Input: part model. Units: mm. Frame: model coordinates. Give positions to 0.01 mm unless a question says otherwise; leave off trailing zeros. Loops run counter-clockwise (first coordinate to the right, second up) from the corner with the lowest first, then second, coordinate; pieces in that order, holes last. Notation, with made-up numbers: (67, -17) - (91, -17) arc R16 cw to (91, 11) - close; hole circle Ø2 at (16, 69.5). An arc over 180 degrees is marked (long way). One line per item, written item: value.
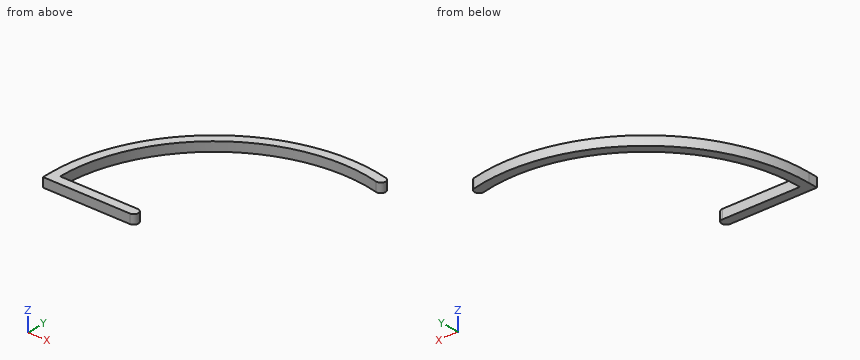
from build123d import *

# Parameters (mm, degrees)
BOSS_EXTRUDE1_DEPTH = 5


with BuildPart() as part:
    # Sketch1 → Boss-Extrude1 (new, symmetric)
    with BuildSketch(Plane.XY):
        with BuildLine():
            Line((552.821544179, 848.961112624), (459.088326812, 848.961112624))
            Line((459.088326812, 848.961112624), (459.088326812, 858.961112624))
            ThreePointArc((459.088326812, 858.961112624), (525.634918269, 996.884166681), (675.00895728, 1030.627523725))
            ThreePointArc((675.00895728, 1030.627523725), (678.753172827, 1024.629119776), (672.754768877, 1020.884904229))
            ThreePointArc((672.754768877, 1020.884904229), (531.858185738, 989.056590938), (469.088326812, 858.961112624))
            Line((469.088326812, 858.961112624), (552.821544179, 858.961112624))
            ThreePointArc((552.821544179, 858.961112624), (557.821544179, 853.961112624), (552.821544179, 848.961112624))
        make_face()
    extrude(amount=BOSS_EXTRUDE1_DEPTH, both=True)


solid = part.part
Item 1: Pin query (flat end, axial travel): P1, Ø1, axis at y = 982.5, z = -0.5, coming from the +X side; P2, Ø3, axis at x = 525.5, z = -2, coming from the +Y side; P3, Ø4, axis at y = 966, z = 3, coming from the +X side. Return the tip coordinate at first contact, or that it passes through.
Verdict:
P1: stops at x = 524.67
P2: stops at y = 997.96
P3: stops at x = 509.86
Item 2: Section A-A, the plane x = 495.5. Output: boundary loops of the cut face in (y, z), and give its area (3 significant figures).
Verdict:
outline: (848.96, -5) - (858.96, -5) - (858.96, 5) - (848.96, 5) - close; (948.86, -5) - (966.23, -5) - (966.23, 5) - (948.86, 5) - close
area: 274 mm^2
Item 3: Section C-C, the plane x = 530. Output: boundary loops of the cut face in (y, z).
Verdict:
outline: (848.96, -5) - (858.96, -5) - (858.96, 5) - (848.96, 5) - close; (987.56, -5) - (1000.24, -5) - (1000.24, 5) - (987.56, 5) - close
Item 4: Section B-B, the plane z = 1. Output: boundary loops of the cut face in (x, y), and give its area (3 significant figures).
Verdict:
outline: (459.09, 848.96) - (552.82, 848.96) arc R5 ccw to (552.82, 858.96) - (469.09, 858.96) arc R166.2 cw to (672.75, 1020.88) arc R5 ccw to (675.01, 1030.63) arc R176.2 ccw to (459.09, 858.96) - close
area: 4,090 mm^2
Item 5: Section D-D, the plane y = 958.5. Output: boundary loops of the cut face in (x, z).
Verdict:
outline: (489.9, -5) - (502.19, -5) - (502.19, 5) - (489.9, 5) - close
Item 6: Material intervals for L1, parallel to Y at x = 533, z = 4; L2, parallel to Y at x = 637.5, z = -1.25; L3, parallel to Y at x = 516, z = 0.25, sorted ascending.
Verdict:
L1: y = 848.96 to 858.96, 989.96 to 1002.43
L2: y = 1025.15 to 1035.15
L3: y = 848.96 to 858.96, 974.69 to 988.64
